Source: CAD feature listing. Evaluate the final solid. Frame: model axes, mm. A direction names the side the tool comes from. Give positions to 0.01 mm unless a question says otherwise; leave off trailing zeros. Loops run counter-clockwise (first coordinate to the right, second up) from the corner with the lowest first, then second, coordinate; pieces in that order, holes last. Notation, with made-up numbers: (-9, 15) -> (50, 15) arc R23 ccw to (50, 41) -> close; hole circle Ø7 at (33, 46). An arc over 180 degrees is marked (long way). Return JSON: item names as keys, results as strings. Group by question number.
```python
from build123d import *

# Parameters (mm, degrees)
CROQUIS1_W                 = 21
CROQUIS1_H                 = 36
SALIENTE_EXTRUIR1_DEPTH    = 5
CROQUIS2_OUTSIDE_W         = 31.396
CROQUIS2_OUTSIDE_H         = 46.396
CROQUIS2_OUTSIDE_W_2       = 7.048063548
CROQUIS2_OUTSIDE_H_2       = 7
CORTAR_EXTRUIR1_DEPTH      = 7
CORTAR_EXTRUIR1_DEPTH_BACK = 4
CROQUIS3_W                 = 7
CROQUIS3_H                 = 4.02225483
SALIENTE_EXTRUIR2_DEPTH    = 3
CROQUIS4_W                 = 5.679391124
CROQUIS4_H                 = 1.977645124
CORTAR_EXTRUIR2_DEPTH      = 3
CROQUIS5_W                 = 5.67716457
CROQUIS5_H                 = 2.946376549
CORTAR_EXTRUIR3_DEPTH      = 6
REDONDEO1_R                = 2
CROQUIS7_R                 = 1.5
CORTAR_EXTRUIR4_DEPTH      = 10
CROQUIS8_R                 = 1.5
CORTAR_EXTRUIR5_DEPTH      = 10
CROQUIS9_R                 = 0.798287554
CORTAR_EXTRUIR6_DEPTH      = 10
MATRIZL1_COUNT             = 8
MATRIZL1_PITCH             = 3


with BuildPart() as part:
    # Croquis1 → Saliente-Extruir1 (new body)
    with BuildSketch(Plane(origin=(0, 0, 0), x_dir=(1, 0, 0), z_dir=(0, 1, 0))):
        Rectangle(CROQUIS1_W, CROQUIS1_H)
    extrude(amount=SALIENTE_EXTRUIR1_DEPTH)

    # Croquis2 outside → Cortar-Extruir1 (cut, two sides)
    with BuildSketch(Plane(origin=(0, 5, 0), x_dir=(1, 0, 0), z_dir=(0, 1, 0))) as cortar_extruir1_sk:
        Rectangle(CROQUIS2_OUTSIDE_W, CROQUIS2_OUTSIDE_H)
        with Locations((-6.975968226, 5.5)):
            Rectangle(CROQUIS2_OUTSIDE_W_2, CROQUIS2_OUTSIDE_H_2, mode=Mode.SUBTRACT)
    extrude(amount=CORTAR_EXTRUIR1_DEPTH, mode=Mode.SUBTRACT)
    extrude(cortar_extruir1_sk.sketch, amount=-CORTAR_EXTRUIR1_DEPTH_BACK, mode=Mode.SUBTRACT)

    # Croquis3 → Saliente-Extruir2 (add)
    with BuildSketch(Plane(origin=(0, 1, 0), x_dir=(1, 0, 0), z_dir=(0, 1, 0))):
        with Locations((0, 15.988872585)):
            Rectangle(CROQUIS3_W, CROQUIS3_H)
    extrude(amount=SALIENTE_EXTRUIR2_DEPTH)

    # Croquis4 → Cortar-Extruir2 (cut)
    with BuildSketch(Plane(origin=(0, 0, -18), x_dir=(-1, 0, 0), z_dir=(0, 0, -1))):
        with Locations((0.114094911, 2.309841815)):
            Rectangle(CROQUIS4_W, CROQUIS4_H)
    extrude(amount=-CORTAR_EXTRUIR2_DEPTH, mode=Mode.SUBTRACT)

    # Croquis5 → Cortar-Extruir3 (cut)
    with BuildSketch(Plane.ZY.offset(10.5)):
        with Locations((-5.467429763, 2.848675026)):
            Rectangle(CROQUIS5_W, CROQUIS5_H)
    extrude(amount=-CORTAR_EXTRUIR3_DEPTH, mode=Mode.SUBTRACT)

    # Redondeo1
    redondeo1_edges = [part.edges().sort_by_distance(p)[0] for p in [
        (-10.5, 0.5, -18),
        (10.5, 0.5, -18),
        (10.5, 0.5, 18),
        (-10.5, 0.5, 18),
    ]]
    fillet(redondeo1_edges, radius=REDONDEO1_R)

    # Croquis7 → Cortar-Extruir4 (cut)
    with BuildSketch(Plane(origin=(0, 1, 0), x_dir=(1, 0, 0), z_dir=(0, 1, 0))):
        with Locations((-8.47455652, 15.912213441)):
            Circle(CROQUIS7_R)
    extrude(amount=-CORTAR_EXTRUIR4_DEPTH, mode=Mode.SUBTRACT)

    # Croquis8 → Cortar-Extruir5 (cut)
    with BuildSketch(Plane(origin=(0, 1, 0), x_dir=(1, 0, 0), z_dir=(0, 1, 0))):
        with Locations((8.231076472, 15.912213441)):
            Circle(CROQUIS8_R)
        with Locations((-8.47455652, -15.850727458)):
            Circle(CROQUIS8_R)
        with Locations((8.231076472, -15.850727458)):
            Circle(CROQUIS8_R)
    extrude(amount=-CORTAR_EXTRUIR5_DEPTH, mode=Mode.SUBTRACT)

    # Croquis9 → Cortar-Extruir6 (cut)
    with BuildSketch(Plane(origin=(0, 1, 0), x_dir=(1, 0, 0), z_dir=(0, 1, 0))):
        with Locations((9.121120171, -10.985155237)):
            Circle(CROQUIS9_R)
    cortar_extruir6 = extrude(amount=-CORTAR_EXTRUIR6_DEPTH, mode=Mode.SUBTRACT)

    # MatrizL1: Cortar-Extruir6 ×8
    with Locations(*[(0, 0, -i * MATRIZL1_PITCH) for i in range(1, MATRIZL1_COUNT)]):
        add(cortar_extruir6, mode=Mode.SUBTRACT)


solid = part.part
```
1) Contact query for flat-ended pins moving along their axis: P1, Ø2, axis at x = -8, y = 4.5, coming from the +Z side; P2, Ø2.5, axis at x = -6.5, y = 2.5, coming from the -Z side; P3, Ø3, axis at x = -5, z = 7, coming from the +Y side; P4, Ø1.4, axis at x = 9.12, z = 7.99, coming from the -Y side. Output: stop coordinate, or through.
2) Reachability of faces 1 (the face through (-8, 3, -8.306)), 2 (the face through (-9.93, 0.51, -17.4)), 3 (the face through (2.726, 2, -17)) from +Z, -Z, +X, -X, +Y, -Y: full face, straight path, thin tool, end or side. Return the list, or none.
3) Cut plane D-D on z = 0.5. Return loops of the section in (x, y).
4) Cut plane C-C on y = 0.65. Count the separate pieces of the cut face and the enclosed holes in it, then the cut area to 3 significant figures.
5) Material intervals for line 1 (Z direction, x = -6.5, y = 2.4); line 2 (Z direction, x = 8.25, y = 0.25); line 3 (X direction, y = 0.65, z = -10), sorted ascending.
6) Cut plane B-B on x = -1.75. Return loops of the section in (y, z).
7) Mould query, pull axis Y, two halves, no side actions, for faces 4 (the face through (0, 1.321, -17)), 5 (the face through (3.5, 2, -16)), 6 (the face through (-7, 5, -6)). Classes: released by +Y, released by -Y, zero draft, split by the parting line, or undercut.
8) Cut plane A-A on y = 2.5. Return loops of the section in (x, z).
Calculated:
{
 "1": {"P1": "z = -2", "P2": "z = -9", "P3": "y = 1", "P4": "through"},
 "2": {"face 1": "-X", "face 2": "-Z, -X, +Y, -Y", "face 3": "-Z"},
 "3": {"outline": "(-10.5, 0) -> (10.5, 0) -> (10.5, 1) -> (-10.5, 1) -> close"},
 "4": {"separate pieces": "1", "enclosed holes": "12", "area": "708 mm2"},
 "5": {"line 1": "-9 to -8.31, -2.63 to -2", "line 2": "-18 to -17.41, -14.41 to 14.35, 17.35 to 18", "line 3": "-10.5 to 8.32, 9.92 to 10.5"},
 "6": {"outline": "(0, -18) -> (1.32, -18) -> (1.32, -15) -> (3.3, -15) -> (3.3, -18) -> (4, -18) -> (4, -13.98) -> (1, -13.98) -> (1, 18) -> (0, 18) -> close"},
 "7": {"face 4": "undercut", "face 5": "zero draft", "face 6": "released by +Y"},
 "8": {"outline": "(-10.5, -9) -> (-3.45, -9) -> (-3.45, -2) -> (-10.5, -2) -> (-10.5, -2.63) -> (-4.5, -2.63) -> (-4.5, -8.31) -> (-10.5, -8.31) -> close; (-3.5, -18) -> (-2.95, -18) -> (-2.95, -15) -> (2.73, -15) -> (2.73, -18) -> (3.5, -18) -> (3.5, -13.98) -> (-3.5, -13.98) -> close"}
}
